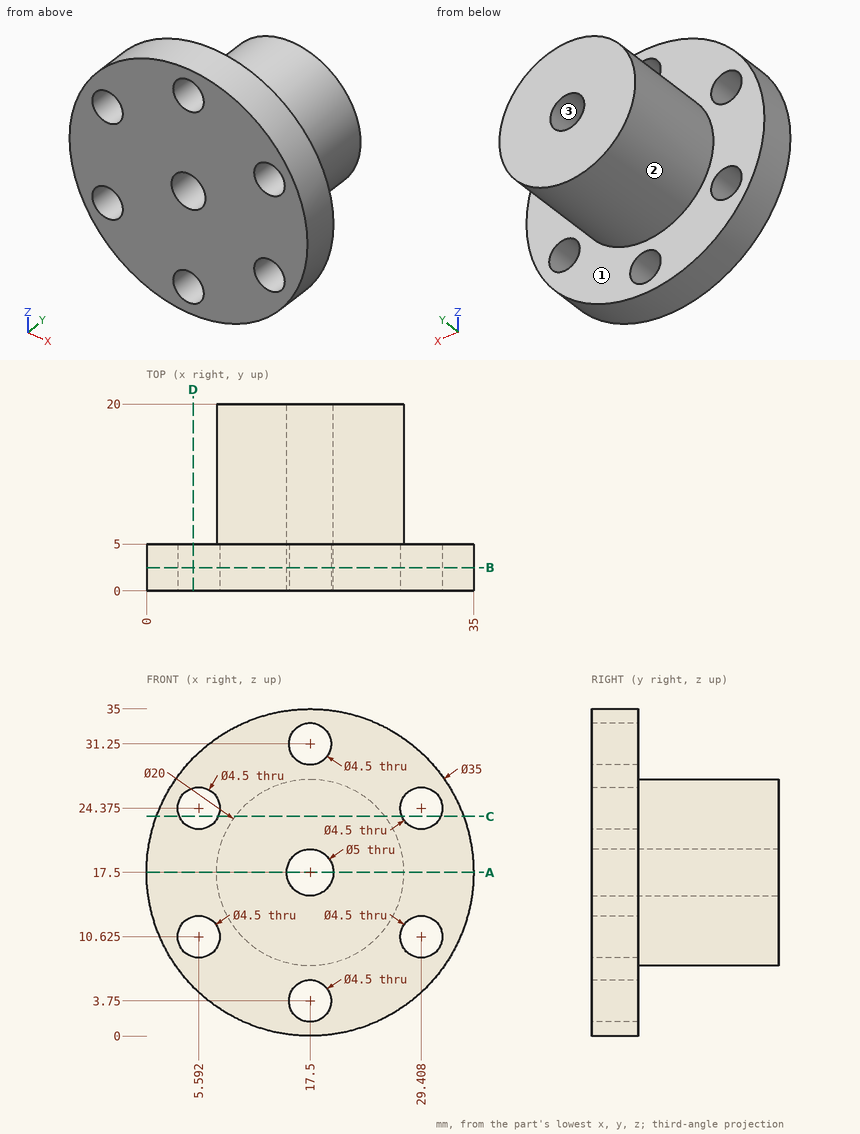
The drawing under review shows one solid part. Ordinate dimensions are in mm from its lowest x, y, z. Round coordinates to 2 decimals unless told otherwise and drop trailing zeros. Order: outer loops, then holes, each group sorted by start corner. A loop starts at its lowest first (then second) coordinate and runs counter-clockwise, first axis right, second up. Notation, with made-up numbers: (83, -32.75) - (123, -32.75) arc R20 cw to (123, 0.25) - close; hole circle Ø11 at (60, 88). An arc over 180 degrees is marked (long way). Return JSON: item names as keys, results as strings.
Q1. For pin 1 Ø3 at (y, z) = (14, 13.5) entering from -X; pin 2 Ø7 at (x, z) = (5.59, 24.38) entering from +Y; pin 3 Ø6 at (x, z) = (20.5, 15) entering from -Y; pin 4 Ø2 at (x, y) = (23.5, 17.5) entering from -Z, all flat-tipped, find the tip position at first contact; note any pin that passes through.
Computed values:
{"pin 1": "stops at x = 7.82", "pin 2": "stops at y = 5", "pin 3": "stops at y = 0", "pin 4": "stops at z = 8.84"}
Q2. Consider section B-B on y = 2.5. Write out the cut boundary in (x, z) (3 decimals), plus the area to 3 significant figures.
Computed values:
{"outline": "circle Ø35 at (17.5, 17.5); hole circle Ø4.5 at (5.592, 10.625); hole circle Ø4.5 at (5.592, 24.375); hole circle Ø5 at (17.5, 17.5); hole circle Ø4.5 at (17.5, 3.75); hole circle Ø4.5 at (17.5, 31.25); hole circle Ø4.5 at (29.408, 10.625); hole circle Ø4.5 at (29.408, 24.375)", "area": "847 mm2"}
Q3. Consider section C-C on z = 23.5. Write out the cut boundary in (x, y) (1 decimal).
Computed values:
{"outline": "(1.1, 0) - (3.5, 0) - (3.5, 5) - (1.1, 5) - close; (7.7, 0) - (27.3, 0) - (27.3, 5) - (25.5, 5) - (25.5, 20) - (9.5, 20) - (9.5, 5) - (7.7, 5) - close; (31.5, 0) - (33.9, 0) - (33.9, 5) - (31.5, 5) - close"}
Q4. Consider section D-D on x = 5. Write out the cut boundary in (y, z).
Computed values:
{"outline": "(0, 5.25) - (5, 5.25) - (5, 8.45) - (0, 8.45) - close; (0, 12.8) - (5, 12.8) - (5, 22.2) - (0, 22.2) - close; (0, 26.55) - (5, 26.55) - (5, 29.75) - (0, 29.75) - close"}
Q5. Consider section A-A on z = 17.5. Write out the cut boundary in (x, y), plus the area to 3 significant figures.
Computed values:
{"outline": "(0, 0) - (15, 0) - (15, 20) - (7.5, 20) - (7.5, 5) - (0, 5) - close; (20, 0) - (35, 0) - (35, 5) - (27.5, 5) - (27.5, 20) - (20, 20) - close", "area": "375 mm2"}
Q6. The part is to be moulded in two halves that separate along X. For the marked faces 1, 2 and 3, say which applies: pulls with the +X half, pulls with the -X half, needs draft (parallel to the pull), parting line crosses it, or undercut.
Computed values:
{"face 1": "needs draft", "face 2": "parting line crosses it", "face 3": "undercut"}
Q7. Wall thickness on L1, parallel to X at y = 4, z = 23; L2, parallel to X at y = 4, z = 17.5; L3, parallel to Y at x = 22, z = 7.5: over which ranges is each line inside the solid? List them lowest first. Write a range as [from, to].
Computed values:
{"L1": "x = [0.89, 3.81], [7.37, 27.63], [31.19, 34.11]", "L2": "x = [0, 15], [20, 35]", "L3": "y = [0, 5]"}
